Geometry check sheet. Reference: the model listing, model coordinates, mm. A direction names the side the tool comes from. Coordinates: 2 decimals unless noted, no trailing zeros. Order: outer loops, then holes, each group sorted by start corner. A loop starts at its lowest first (then second) coordinate and runs counter-clockwise, first axis right, second up. Notation, with made-up numbers: (38.25, 68.5) - (58.25, 68.5) arc R23 ccw to (58.25, 82.5) - close; hole circle Ø7 at (19, -31.75). An arc over 180 degrees is marked (long way). Return JSON: item names as keys, results as strings. Group by question number.
Item 1: Tool access check on faces 4 (the flat face through (-5.353, 3.176, -20.14)), 5 (the flat face through (-7.565, 1, -40)), 6 (the flat face through (-7.565, 1, 0)), 7 (the flat face through (-26, 0, -1)), 8 (the cylindrical face through (-4.96, 2.08, 19.86)). Record the directions out of +Z, -Z, +X, -X, +Y, -Y that give a thin tool (end or side, any length) a straight path to the whole face; none if there is none.
Item 2: Section check A-A on y = 4.5. Enter the section's corners in (x, z).
Item 3: Section check B-B on z = 24. Enter the section's corners in (x, y).
Item 4: Draft check along Y on faces 1 (the conical face through (-37, 0.16, -2.13)), 2 (the flat face through (-5.353, 3.176, 19.86)), 3 (the flat face through (4.5, 4.3, 10)). Enter one of: pulls with the +Y half, pulls with the -Y half, needs draft (parallel to the pull), parting line crosses it, or undercut.
Item 5: Section check C-C on z = -40. Enter the section's corners in (x, y).
Item 6: Section check D-D on x = -11.5. Enter the section's corners in (y, z).
Item 7: Gauge pin test, flat ends, axial feed: pin 1 (7 mm diameter, centred on x = 0, y = 4.21, fed in from +Z); pin 2 (6 mm diameter, centred on x = -35, z = -18.5, fed in from -Y); pin 3 (7 mm diameter, centred on x = 2.5, y = 1.5, fed in from +Z); pin 4 (7 mm diameter, centred on x = -2.5, y = 3.5, fed in from -Z). Record the tip position at first contact, or that the pin passes through.
Item 8: Scan lines: probe 1 along Z at (x, y) = (-26, 1.5); probe 2 along Z at (x, y) = (3, 0.5); probe 3 along Y at (x, z) = (-33, 18). Record each from-to range of solid material in increasing order.
Autodesk Inventor part; units mm, degrees
ref_plane "YZ Plane" through (0, 0, 0) normal (1, 0, 0) x (0, 1, 0)
ref_plane "XZ Plane" through (0, 0, 0) normal (0, 1, 0) x (-1, 0, 0)
ref_plane "XY Plane" through (0, 0, 0) normal (0, 0, 1) x (1, 0, 0)
sketch "Sketch1" plane through (0, 0, 0) normal (0, 0, 1) x (1, 0, 0)
  line L0 (-44.6809, 2.5) -> (-7.5647, 2.5)
  line L1 (-44.6809, 0) -> (-44.6809, 2.5)
  line L2 (0, 0) -> (0, 19.2246)
  arc A0 (-3.8253, -1.3563) -> (-6.7141, 3.5099) centre (0, 4.2052) ccw
  arc A1 (-2.5687, 0.8193) -> (-4.0285, 2.8511) centre (0, 4.2052) ccw
  arc A2 (-2.5687, 0.8193) -> (-7.5647, 2.5) centre (-7.5647, -5.7659) ccw
  line L3 (-4.0285, 2.8511) -> (-6.7141, 3.5099)
  arc A3 (-3.8253, -1.3563) -> (-8.1904, 0) centre (-8.1904, -7.7027) ccw
  line L4 (-8.1904, 0) -> (-44.6809, 0)
  line L5 (-36.0171, 0) -> (-5.5909, 0)
  line L6 (-5.2801, 0) -> (0, 0)
  point P0 (0, 10.9552)
  point P1 (0, 8.4552)
  dimension "d1" = 2.5
  dimension "d2" = 2.5
  dimension "d3" = 8.5
extrude "Extrusion1" add sketch "Sketch1" along normal mid plane 100 contours L0 A2 A1 L2 A0 A3 L4 L1 | A1 L3 A0 L2
sketch "Sketch2" plane through (-44.6809, 2.5, 50) normal (0, 1, 0) x (1, 0, 0)
  circle A0 centre (20, 90) radius 4
  circle A1 centre (10, 50) radius 4
  circle A2 centre (20, 10) radius 4
  line L0 (0, 100) -> (37.1161, 100)
  line L1 (0, 100) -> (0, 0)
  line L2 (37.1161, 0) -> (0, 0)
  point P0 (44.6809, 50)
  dimension "d6" = 8
  dimension "d7" = 8
  dimension "d8" = 8
  dimension "d9" = 10
  dimension "d10" = 20
  dimension "d11" = 20
  dimension "d12" = 10
  dimension "d13" = 10
  dimension "d14" = 50
extrude "Extrusion2" cut sketch "Sketch2" against normal up to next draft -20
sketch "Sketch3" plane through (-44.6809, 2.5, 50) normal (0, 1, 0) x (1, 0, 0)
  line L0 (37.1161, 0) -> (37.1161, 100)
  line L1 (37.1161, 100) -> (67.1161, 100)
  line L2 (67.1161, 100) -> (67.1161, 80)
  line L3 (67.1161, 80) -> (37.1161, 80)
  line L4 (37.1161, 80) -> (37.1161, 100)
  line L5 (37.1161, 60) -> (67.1161, 60)
  line L6 (67.1161, 60) -> (67.1161, 40)
  line L7 (67.1161, 40) -> (37.1161, 40)
  line L8 (37.1161, 40) -> (37.1161, 60)
  line L9 (37.1161, 0) -> (0, 0)
  line L10 (37.1161, 0) -> (70.6977, 0)
  line L11 (70.6977, 0) -> (70.6977, 20)
  line L12 (70.6977, 20) -> (37.1161, 20)
  line L13 (37.1161, 20) -> (37.1161, 0)
  point P0 (44.6809, 50)
  point P1 (37.1161, 20)
  dimension "d17" = 20
  dimension "d18" = 30
  dimension "d19" = 20
  dimension "d20" = 20
  dimension "d21" = 20
extrude "Extrusion3" cut sketch "Sketch3" against normal mid plane 100
properties part number "Hinge1" material "Stainless Steel"
Computed:
{
 "1": {"face 4": "+Z, -Z, -X", "face 5": "-Z, +X, +Y, -Y", "face 6": "+X, +Y, -Y", "face 7": "+Z, -Z, -X, -Y", "face 8": "+Z, -Z"},
 "2": {"outline": "(-6.74, -30) - (-4.24, -30) - (-4.24, -10) - (-6.74, -10) - close; (-6.74, 10) - (-4.24, 10) - (-4.24, 30) - (-6.74, 30) - close; (4.24, -30) - (6.74, -30) - (6.74, -10) - (4.24, -10) - close; (4.24, 10) - (6.74, 10) - (6.74, 30) - (4.24, 30) - close"},
 "3": {"outline": "(-44.68, 0) - (-8.19, 0) arc R7.7 cw to (-3.83, -1.36) arc R6.75 ccw (long way) to (-6.71, 3.51) - (-4.03, 2.85) arc R4.25 cw (long way) to (-2.57, 0.82) arc R8.27 ccw to (-7.56, 2.5) - (-44.68, 2.5) - close"},
 "4": {"face 1": "pulls with the +Y half", "face 2": "undercut", "face 3": "needs draft"},
 "5": {"outline": "(-44.68, 0) - (-27.77, 0) - (-28.68, 2.5) - (-44.68, 2.5) - close; (-21.59, 0) - (-8.19, 0) arc R7.7 cw to (-7.56, -0.03) - (-7.56, 2.5) - (-20.68, 2.5) - close"},
 "6": {"outline": "(0, -50) - (2.5, -50) - (2.5, 50) - (0, 50) - close"},
 "7": {"pin 1": "passes through", "pin 2": "stops at y = 0", "pin 3": "stops at z = 30", "pin 4": "stops at z = -30"},
 "8": {"probe 1": "z = -50 to -43.39, -36.61 to 36.61, 43.39 to 50", "probe 2": "z = -30 to -10, 10 to 30", "probe 3": "y = 0 to 2.5"}
}
